Geometry check sheet. Reference: the model listing, model coordinates, mm. A direction names the side the tool comes from. Coordinates: 2 decimals unless noted, no trailing zeros. Write each loop counter-clockwise with the first axis right and the second up, starting at its lowest first coordinate (ties: lowest second). Pieces come first, ordered by that corner, then holes. Notation, with made-up numbers: (65, 70.5) -> (77, 70.5) arc R34 ccw to (77, 106.5) -> close; hole circle Ø10 at (-16, -26). An arc over 180 degrees is marked (long way). One line per question, with ' | ' between items.
from build123d import *

# Parameters (mm, degrees)
BOSS_EXTRUDE1_DEPTH = 38.1
SKETCH2_W           = 38.1
SKETCH2_H           = 8.128
CUT_EXTRUDE1_DEPTH  = 458.2


with BuildPart() as part:
    # Sketch1 → Boss-Extrude1 (new body)
    with BuildSketch(Plane(origin=(0, 0, 0), x_dir=(1, 0, 0), z_dir=(0, 1, 0))):
        with BuildLine():
            Line((-228.6, 457.2), (-76.2, 457.2))
            Line((-76.2, 457.2), (-76.2, 431.052293811))
            ThreePointArc((-76.2, 431.052293811), (222.015661474, -77.313424673), (-228.6, -457.2))
            Line((-228.6, -457.2), (-228.6, 457.2))
        make_face()
    extrude(amount=BOSS_EXTRUDE1_DEPTH)

    # Sketch2 → Cut-Extrude1 (cut, through all)
    with BuildSketch(Plane.ZY.offset(228.6)):
        with Locations((457.2, 19.05)):
            Rectangle(SKETCH2_W, SKETCH2_H)
        with Locations((-457.2, 19.05)):
            Rectangle(SKETCH2_W, SKETCH2_H)
    extrude(amount=-CUT_EXTRUDE1_DEPTH, mode=Mode.SUBTRACT)


solid = part.part
1. Cross-section at C-C on z = -377. Record the boundary of the cut face in (x, y).
Worked answers:
outline: (-228.6, 0) -> (30.06, 0) -> (30.06, 38.1) -> (-228.6, 38.1) -> close
2. Material ranges on line 1 (Z direction, x = -175, y = 18); line 2 (Z direction, x = 102.5, y = 34) (3 decimals); line 3 (X direction, y = 13.5, z = 83), recorded low to high. Write a range as from..to.
Worked answers:
line 1: -438.15..438.15 | line 2: -315.285..315.285 | line 3: -228.6..221
3. Go/stop test with flat-tipped pins: P1, Ø4, axis at x = -150.5, y = 19, coming from the -Z side; P2, Ø5, axis at y = 12, z = -234, coming from the +X side; P3, Ø12, axis at x = -108.5, y = 17.5, coming from the -Z side; P4, Ø6, axis at y = 25.5, z = -284.5, coming from the +X side. Record where each tip stops, or that it passes through.
Worked answers:
P1: z = -438.15 | P2: x = 165.66 | P3: z = -457.2 | P4: x = 131.66
4. Cross-section at B-B on x = -87. Record the boundary of the cut face in (y, z), and give its area (3 significant figures).
Worked answers:
outline: (0, -457.2) -> (14.99, -457.2) -> (14.99, -438.15) -> (23.11, -438.15) -> (23.11, -457.2) -> (38.1, -457.2) -> (38.1, 434.72) -> (0, 434.72) -> close | area: 33,800 mm²
5. Cross-section at A-A on y = 7.5. Record the boundary of the cut face in (x, z), and give its area (3 significant figures).
Worked answers:
outline: (-228.6, -457.2) -> (-76.2, -457.2) -> (-76.2, -431.05) arc R457.2 ccw to (-228.6, 457.2) -> close | area: 330,000 mm²
6. Tool access check on faces 5 (the face through (-76.2, 14.5, -444.3)), 6 (the face through (-48, 0, -6)), 7 (the face through (-179, 23.114, 445)), 8 (the face through (-153, 23.114, -448)). Record the directions out of +Z, -Z, +X, -X, +Y, -Y that give a thin tool (end or side, any length) a straight path to the whole face; none if there is none.
Worked answers:
face 5: -Z, +X, +Y, -Y | face 6: +Z, -Z, +X, -X, -Y | face 7: +Z, +X, -X | face 8: -Z, +X, -X
7. Mould release check, pull along Y, two halves, no side actions. Record for faces 1 (the face through (-48, 38.1, -6)), 2 (the face through (-153, 14.986, -448)), 3 (the face through (-228.6, 19, 6)), 4 (the face through (-179, 14.986, 445)): released by +Y, released by -Y, zero draft, split by the parting line, or undercut.
Worked answers:
face 1: released by +Y | face 2: undercut | face 3: zero draft | face 4: undercut
